Verification items for the finished model (mm, model axes). Face numbers are marked on the shaded views. A direction names the side the tool comes from. Round coordinates to 2 decimals unless told otherwise and drop trailing zeros. Order: outer loops, then holes, each group sorted by start corner. A loop starts at its lowest first (then second) coordinate and runs counter-clockwise, first axis right, second up. Notation, with made-up numbers: (-23.5, -20.5) -> (9.5, -20.5) arc R14 cw to (9.5, 0.5) -> close; hole circle Ø6 at (-35, 32.25). An arc over 180 degrees is marked (long way). Write item = value, one per line. Start each with the question number.
from build123d import *

# Parameters (mm, degrees)
F0_W     = 101.6
F0_H     = 101.6
F1_DEPTH = 3
F2_DEPTH = 25
F3_R     = 2


with BuildPart() as f1:
    # F0 (on Top) → F1 (new body)
    with BuildSketch(Plane.XY):
        Polygon((-50.8, -50.8), (-50.8, 50.8), (-74.547097, 29.664359), (-74.547097, -32.537002), align=None)
        Rectangle(F0_W, F0_H)
        Polygon((76.217584, 26.386153), (50.8, 50.8), (50.8, -50.8), (76.217584, -37.332729), align=None)
    extrude(amount=F1_DEPTH)

    # F0 (on Top) → F2 (join)
    with BuildSketch(Plane.XY):
        Polygon((-51.30187, 54.977957), (-77.688023, 31.450987), (-77.688023, -35.208765), (-50.8, -54.43063), (50.8, -54.43063), (79.613134, -39.051957), (79.613134, 27.056271), (51.138487, 54.814577), align=None)
        Polygon((-74.547097, 29.664359), (-50.8, 50.8), (50.8, 50.8), (76.217584, 26.386153), (76.217584, -37.332729), (50.8, -50.8), (-50.8, -50.8), (-74.547097, -32.537002), align=None, mode=Mode.SUBTRACT)
    extrude(amount=F2_DEPTH)

    # F3
    f3_edges = [f1.edges().sort_by_distance(p)[0] for p in [
        (-50.8, -54.43063, 12.5),
        (-77.688023, -35.208765, 12.5),
        (50.8, -54.43063, 12.5),
        (79.613134, -39.051957, 12.5),
        (79.613134, 27.056271, 12.5),
        (51.138487, 54.814577, 12.5),
        (-51.30187, 54.977957, 12.5),
        (-77.688023, 31.450987, 12.5),
    ]]
    fillet(f3_edges, radius=F3_R)


solid = f1.part
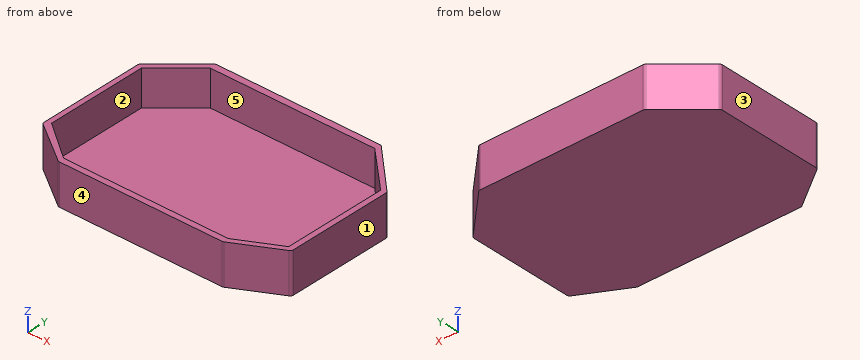
(1) Draft check along Y on the marked faces 3, 4 and 5. Enter one of: +Y half, -Y half, draft (parallel to the pull), parting line (faces both ways), or undercut.
(2) Set-up check for the marked faces 1 and 2: record each of +Z, -Z, +X, -X, +Y, -Y from which the full face is reachable in a straight line by a thin tool's end or side.
(3) Cross-section at C-C (x = 67.5). Enter the section's corners in (y, z), and give its area (3 significant figures).
(4) Cross-section at B-B (y = -11). Enter the section's corners in (x, z), and give its area (3 significant figures).
(5) Scan lines: line 1 along Y through (x, z) = (37.5, 7.25); line 2 along X through (y, z) = (-32, 16.25); line 3 along Z through (x, y) = (-70, 21). Record each from-to range of solid material in increasing order. Write a range as from..to.
(6) Depth check by flat-ended pin: pin 1 (6.5 mm diameter, centred on x = -17, z = 19, fed in from +Y); pin 2 (5 mm diameter, centred on x = -52, y = -17, fed in from +Z); pin 3 (1.5 mm diameter, centred on x = 58.5, z = 10, fed in from -Y). Enter the tip coordinate at first touch or a pass-through.
(7) Cross-section at A-A (z = 16.5). Enter the section's corners in (x, y) (3 decimals).
Outcome:
q1.face_3 = draft
q1.face_4 = -Y half
q1.face_5 = undercut
q2.face_1 = +Z, -Z, +X, +Y, -Y
q2.face_2 = +Z
q3.outline = (-45.52, 0) -> (38.86, 0) -> (38.86, 25) -> (34.76, 25) -> (34.76, 3) -> (-41.95, 3) -> (-41.95, 25) -> (-45.52, 25) -> close
q3.area = 422 mm^2
q4.outline = (-77.69, 0) -> (79.61, 0) -> (79.61, 25) -> (76.22, 25) -> (76.22, 3) -> (-74.55, 3) -> (-74.55, 25) -> (-77.69, 25) -> close
q4.area = 616 mm^2
q5.line_1 = -54.43..-50.8, 50.8..54.84
q5.line_2 = -77.69..-74.55, 76.22..79.61
q5.line_3 = 0..3
q6.pin_1 = 54.93
q6.pin_2 = 3
q6.pin_3 = -50.72
q7.outline = (-77.688, -34.18) arc R2 ccw to (-76.851, -35.807) -> (-51.322, -54.058) arc R2 ccw to (-50.159, -54.431) -> (50.3, -54.431) arc R2 ccw to (51.241, -54.195) -> (78.555, -39.617) arc R2 ccw to (79.613, -37.852) -> (79.613, 26.213) arc R2 ccw to (79.009, 27.645) -> (51.72, 54.248) arc R2 ccw to (50.327, 54.816) -> (-50.538, 54.977) arc R2 ccw to (-51.872, 54.47) -> (-77.019, 32.047) arc R2 ccw to (-77.688, 30.555) -> close; hole (-74.547, -32.537) -> (-50.8, -50.8) -> (50.8, -50.8) -> (76.218, -37.333) -> (76.218, 26.386) -> (50.8, 50.8) -> (-50.8, 50.8) -> (-74.547, 29.664) -> close
